```python
from build123d import *

# Parameters (mm, degrees)
CHAMFER1_SIZE = 0.5


with BuildPart() as part:
    # Sketch1 → Revolve1 (revolve)
    with BuildSketch(Plane.XY):
        Polygon((0, 0), (0, 59.9), (-7.3, 59.9), (-7.9, 59.3), (-8.9, 59.3), (-9.5, 59.9), (-14, 59.9), (-15, 59), (-27.6, 59), (-37.6, 49), (-48.1, 49), (-48.1, 45.25), (-48.8, 45.25), (-48.8, 41.5), (-50.8, 41.5), (-50.8, 42.5), (-58.1, 42.5), (-58.1, 41.5), (-59.6, 41.5), (-59.6, 36), (-65.2, 36), (-65.2, 32), (-66.2, 32), (-66.2, 0), align=None)
    revolve(axis=Axis((0, 0, 0), (-1, 0, 0)))

    # Chamfer1
    chamfer1_edges = [part.edges().sort_by_distance(p)[0] for p in [
        (0, -59.9, 0),
    ]]
    chamfer(chamfer1_edges, length=CHAMFER1_SIZE)


solid = part.part
```
Verification items for the finished model (mm, model axes). A direction names the side the tool comes from. Give positions to 0.01 mm unless a question says otherwise; leave off trailing zeros. Loops run counter-clockwise (first coordinate to the right, second up) from the corner with the lowest first, then second, coordinate; pieces in that order, holes last.
1. Go/stop test with flat-tipped pins: pin 1 Ø2 at (y, z) = (-45, -33) entering from -X; pin 2 Ø1 at (x, y) = (-8.5, 26.5) entering from +Z; pin 3 Ø8 at (x, y) = (-56.5, 32.5) entering from -Z. Record where each tip stops, or that it passes through.
2. Section check A-A, the plane x = -25. Enter the section's corners in (y, z), then the cut area to 3 significant figures.
3. Thickness scan on line 1 (X direction, y = -15, z = 30); line 2 (Y direction, x = -13, z = -1); line 3 (X direction, y = -41, z = -19.5). Record the ranges inside material, lowest first.
4. Mould release check, pull along X, two halves, no side actions. Record for faces 4 (the flat face through (-66.2, 0, 0)), 5 (the flat face through (-48.8, 20, 37)), 6 (the cylindrical face through (-48.45, 43.16, -13.59)): released by +X, released by -X, zero draft, split by the parting line, or undercut.
5. Set-up check for faces 1 (the flat face through (-50.8, -9, 41)), 2 (the cylindrical face through (-65.71, -6.94, 31.24)), 3 (the cylindrical face through (-3.948, 57.134, -17.992)): record each of +Z, -Z, +X, -X, +Y, -Y from which the full face is reachable in a straight line by a thin tool's end or side.
Geometry says:
1. pin 1: stops at x = -31.8
1. pin 2: stops at z = 53.3
1. pin 3: stops at z = -31.53
2. outline: circle Ø118 at (0, 0)
2. area: 10,900 mm2
3. line 1: x = -65.2 to 0
3. line 2: y = -59.89 to 59.89
3. line 3: x = -48.1 to 0
4. face 4: released by -X
4. face 5: undercut
4. face 6: zero draft
5. face 1: none
5. face 2: -X
5. face 3: +X, -X
